Design review of the part shown in the three views and the two pictorial views. Dimensions are in mm from the part's minimum x, y and z. Coordinates: 2 decimals unless noted, no trailing zeros. Loops run counter-clockwise (first coordinate to the right, second up) from the corner with the lowest first, then second, coordinate; pieces in that order, holes last. Notation, with made-up numbers: (68, -25) - (99, -25) arc R25 ccw to (99, 7) - close; hole circle Ø8 at (59.5, 87.5). An arc over 180 degrees is marked (long way). One line per question, with ' | ' between items.
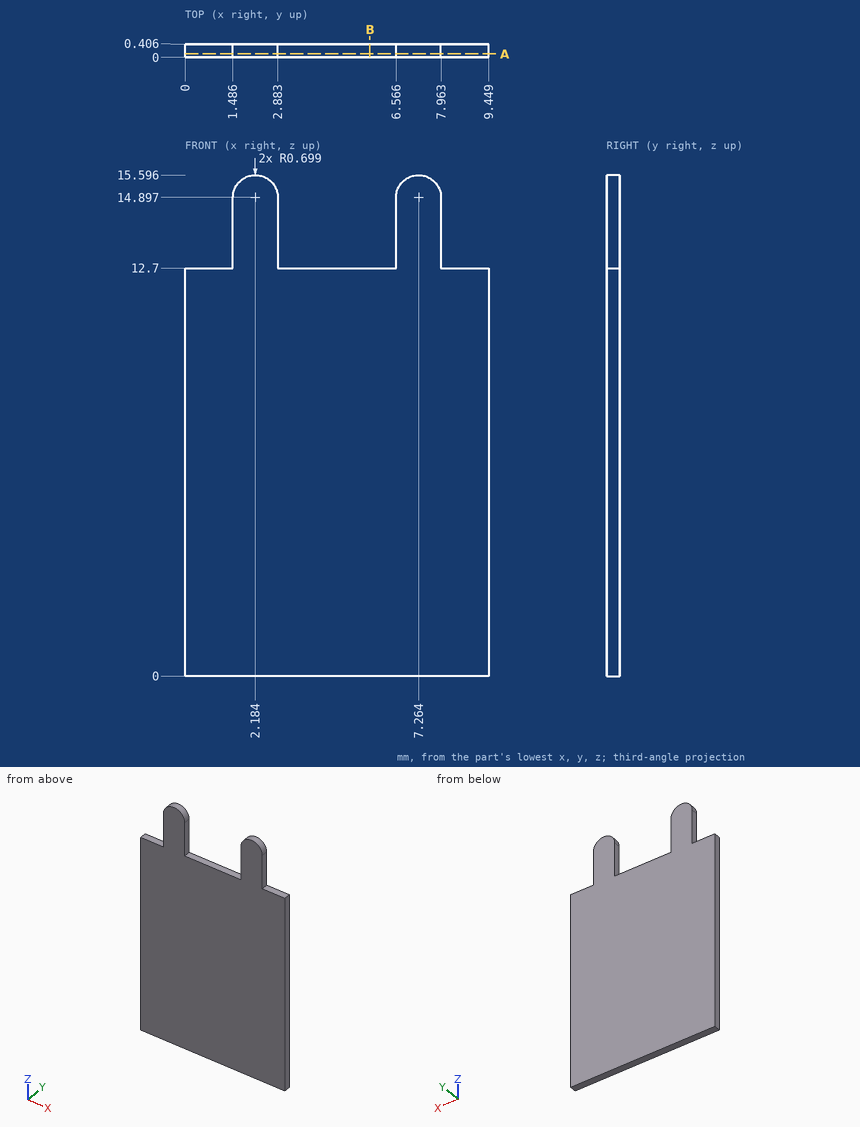
Q1. Take a section at A-A (y = 0.1). Give the boundary of the cut face in (x, z) (1 decimal).
Returned:
outline: (0, 0) - (9.4, 0) - (9.4, 12.7) - (8, 12.7) - (8, 14.9) arc R0.7 ccw to (6.6, 14.9) - (6.6, 12.7) - (2.9, 12.7) - (2.9, 14.9) arc R0.7 ccw to (1.5, 14.9) - (1.5, 12.7) - (0, 12.7) - close
Q2. Take a section at B-B (x = 5.75). Give the boundary of the cut face in (y, z).
Returned:
outline: (0, 0) - (0.41, 0) - (0.41, 12.7) - (0, 12.7) - close
Q3. To check wall thickness, follow line 1 along X through (y, z) = (0.35, 13) (1 decimal); line 2 along Z through (x, y) = (4.25, 0.1); line 3 along Z through (x, y) = (7, 0.1) (1 decimal). State the ranges of each line that lie inside material, in increasing order.
Returned:
line 1: x = 1.5 to 2.9, 6.6 to 8 | line 2: z = 0 to 12.7 | line 3: z = 0 to 15.5
